Autodesk Inventor part; units mm, degrees
ref_plane "YZ Plane" through (0, 0, 0) normal (1, 0, 0) x (0, 1, 0)
ref_plane "XZ Plane" through (0, 0, 0) normal (0, 1, 0) x (-1, 0, 0)
ref_plane "XY Plane" through (0, 0, 0) normal (0, 0, 1) x (1, 0, 0)
sketch "Sketch1" plane through (0, 0, 0) normal (0, 0, 1) x (1, 0, 0)
  line L0 (-8.0095, -1.25) -> (7.9905, -1.25) construction
  line L1 (7.9905, -1.25) -> (7.9905, 1.25) construction
  line L2 (7.9905, 1.25) -> (-8.0095, 1.25) construction
  line L3 (-8.0095, 1.25) -> (-8.0095, -1.25) construction
  line L4 (-8.0095, -1.25) -> (7.9905, 1.25) construction
  line L5 (7.9905, -1.25) -> (-8.0095, 1.25) construction
  circle A0 centre (5.5829, 3.3205) radius 1
  line L6 (-0.0095, 0) -> (-0.0095, 6) construction
  line L7 (-0.0095, 0) -> (-0.0095, -6) construction
  line L8 (-0.0095, 6) -> (-8.0095, 4.75)
  line L9 (-8.0095, 4.75) -> (-8.0095, -4.75)
  line L10 (-8.0095, -4.75) -> (-0.0095, -6)
  line L11 (-0.0095, 6) -> (7.9905, 4.75)
  line L12 (7.9905, 4.75) -> (7.9905, -4.75)
  line L13 (7.9905, -4.75) -> (-0.0095, -6)
  line L14 (7.9905, 4.75) -> (-8.0095, -4.75) construction
  line L15 (-8.0095, 4.75) -> (7.9905, -4.75) construction
  circle A1 centre (-5.6019, 3.3205) radius 1
  line L16 (-8.0095, 0) -> (7.9905, 0) construction
  circle A2 centre (5.5829, -3.3205) radius 1
  circle A3 centre (-5.6019, -3.3205) radius 1
  circle A4 centre (-0.0095, 0) radius 2.54 construction
  line L17 (-0.0095, 0) -> (1.7866, -1.796) construction
  line L18 (-0.0095, 0) -> (-1.8055, -1.796) construction
  line L19 (-0.0095, 0) -> (-1.8055, 1.7961) construction
  circle A5 centre (1.7866, -1.796) radius 0.6
  circle A6 centre (-1.8055, -1.796) radius 0.6
  circle A7 centre (-1.8055, 1.7961) radius 0.6
  point P0 (0, 0)
  point P1 (-0.0095, 0)
  point P2 (-0.0095, 0)
  dimension "d1" = 2.5
  dimension "d2" = 2
  dimension "d3" = 6
  dimension "d4" = 16
  dimension "d5" = 2.8
  dimension "d13" = 5.08
  dimension "d14" = 1.2
extrude "Extrusion2" add sketch "Sketch1" along normal blind 3
sketch "Sketch2" plane through (7.9905, -4.75, 0) normal (1, 0, 0) x (0, 0, -1)
  line L0 (0, 9.5) -> (0, 0)
  arc A0 (-0.7, 5.6) -> (-0.7, 3.9) centre (-0.7, 4.75) ccw
  line L1 (-0.7, 5.6) -> (0, 5.6)
  line L2 (-0.7, 3.9) -> (0, 3.9)
  line L3 (0, 5.6) -> (0, 3.9)
  line L4 (-3, 0) -> (-3, 9.5)
  line L5 (-3, 4.75) -> (-0.7, 4.75) construction
  point P0 (0, 4.75)
  dimension "d11" = 1.7
  dimension "d19" = 0.7
sketch "Sketch3" plane through (0, 0, 0) normal (0, 0, -1) x (-1, 0, 0)
  line L0 (-7.9905, 4.75) -> (-7.9905, -4.75)
  line L1 (8.0095, -4.75) -> (8.0095, 4.75)
  line L2 (-7.9905, 0) -> (8.0095, 0)
  point P0 (0, 0)
sweep "Sweep1" cut profiles "Sketch2" path "Sketch3" path curves L2
properties part number "LED cooling tubing cap 2"
For this review, take the finished solid that the model builds, in its own axes (mm). Coordinates: 2 decimals unless noted, no trailing zeros. Write each loop counter-clockwise with the first axis right and the second up, starting at its lowest first coordinate (ties: lowest second). Pieces come first, ordered by that corner, then holes.
(1) Wall thickness on probe 1 along X at (y, z) = (-3.25, 1); probe 2 along X at (y, z) = (-2, 2.65); probe 3 along Y at (x, z) = (-2, 0.95): over which ranges is each line inside the solid? List them lowest first.
(2) The part is to be moulded in two halves that separate along Y. For faces 1 (the face through (0, -3, 0)), 2 (the face through (4.046, -5.366, 1.479)), 3 (the face through (5.45, 2.33, 1.48)), say which applies: +Y half, -Y half, draft (parallel to the pull), parting line (faces both ways), or undercut.
(3) Add section C-C on z = 2.65. Give the boundary of the cut face in (x, y).
(4) Add section A-A on z = 1.35. Count the separate pieces of the cut face and the enclosed holes in it, then the cut area to 3 significant figures.
(5) For pin 1 Ø0.8 at (x, z) = (-1.5, 0.5) entering from -Y; pin 2 Ø1.5 at (x, z) = (3.5, 1) entering from +Y, all flat-tipped, find the tip position at first contact; note any pin that passes through.
(6) Add section D-D on x = 0.75. Give the boundary of the cut face in (y, z), then the cut area to 3 significant figures.
(7) Add section B-B on y = -3. Give the boundary of the cut face in (x, z), then the cut area to 3 significant figures.
Answer sheet:
1. probe 1: x = -8.01 to -6.6, -4.6 to 4.59, 6.58 to 7.99
1. probe 2: x = -8.01 to -2.37, -1.24 to 1.22, 2.35 to 7.99
1. probe 3: y = -5.69 to -2.36, -1.23 to -0.81, 0.81 to 1.23, 2.36 to 5.69
2. face 1: draft
2. face 2: -Y half
2. face 3: undercut
3. outline: (-8.01, -4.75) - (-0.01, -6) - (7.99, -4.75) - (7.99, 4.75) - (-0.01, 6) - (-8.01, 4.75) - close; hole circle Ø2 at (-5.6, -3.32); hole circle Ø2 at (-5.6, 3.32); hole circle Ø1.2 at (-1.81, -1.8); hole circle Ø1.2 at (-1.81, 1.8); hole circle Ø1.2 at (1.79, -1.8); hole circle Ø2 at (5.58, -3.32); hole circle Ø2 at (5.58, 3.32)
4. separate pieces: 2
4. enclosed holes: 7
4. area: 139 mm2
5. pin 1: stops at y = -5.83
5. pin 2: stops at y = 5.57
6. outline: (-5.88, 0) - (-0.85, 0) - (-0.85, 0.7) arc R0.85 cw to (0.85, 0.7) - (0.85, 0) - (5.88, 0) - (5.88, 3) - (-5.88, 3) - close
6. area: 33.0 mm2
7. outline: (-8.01, 0) - (-6.55, 0) - (-6.55, 3) - (-8.01, 3) - close; (-4.65, 0) - (4.64, 0) - (4.64, 3) - (-4.65, 3) - close; (6.53, 0) - (7.99, 0) - (7.99, 3) - (6.53, 3) - close
7. area: 36.6 mm2
